from build123d import *

# Parameters (mm, degrees)
BOSS_EXTRUDE1_DEPTH                 = 31.75
F_3_32_0_09375_DIAMETER_HOLE1_D     = 2.38125
F_3_32_0_09375_DIAMETER_HOLE1_DEPTH = 25.4
F_3_32_0_09375_DIAMETER_HOLE1_TIP   = 0.715399675
F_10_CLEARANCE_HOLE1_D              = 5.6134
F_10_CLEARANCE_HOLE1_DEPTH          = 25.4
F_10_CLEARANCE_HOLE1_TIP            = 1.686435499
FILLET1_R                           = 2.54


with BuildPart() as part:
    # Sketch1 → Boss-Extrude1 (new body)
    with BuildSketch(Plane.XY):
        Polygon((0, 0), (0, 19.05), (-3.175, 19.05), (-3.175, 3.175), (-19.05, 3.175), (-19.05, 0), align=None)
    extrude(amount=BOSS_EXTRUDE1_DEPTH)

    # 3/32 (0.09375) Diameter Hole1
    with Locations(Plane(origin=(0, 0, 0), x_dir=(0, 0, -1), z_dir=(1, 0, 0))):
        with Locations((-3.175, 0.0889)):
            Hole(F_3_32_0_09375_DIAMETER_HOLE1_D / 2, depth=F_3_32_0_09375_DIAMETER_HOLE1_DEPTH)
            with Locations((0, 0, -(F_3_32_0_09375_DIAMETER_HOLE1_DEPTH + F_3_32_0_09375_DIAMETER_HOLE1_TIP / 2))):  # 118° drill point
                Cone(0, F_3_32_0_09375_DIAMETER_HOLE1_D / 2, F_3_32_0_09375_DIAMETER_HOLE1_TIP, mode=Mode.SUBTRACT)

    # #10 Clearance Hole1
    with Locations(Plane(origin=(0, 3.175, 0), x_dir=(1, 0, 0), z_dir=(0, 1, 0))):
        with Locations((-11.1125, -26.9875), (-11.1125, -4.7625)):
            Hole(F_10_CLEARANCE_HOLE1_D / 2, depth=F_10_CLEARANCE_HOLE1_DEPTH)
            with Locations((0, 0, -(F_10_CLEARANCE_HOLE1_DEPTH + F_10_CLEARANCE_HOLE1_TIP / 2))):  # 118° drill point
                Cone(0, F_10_CLEARANCE_HOLE1_D / 2, F_10_CLEARANCE_HOLE1_TIP, mode=Mode.SUBTRACT)

    # Fillet1
    fillet1_edges = [part.edges().sort_by_distance(p)[0] for p in [
        (-1.5875, 19.05, 31.75),
        (-19.05, 1.5875, 31.75),
        (-19.05, 1.5875, 0),
        (-1.5875, 19.05, 0),
    ]]
    fillet(fillet1_edges, radius=FILLET1_R)


solid = part.part
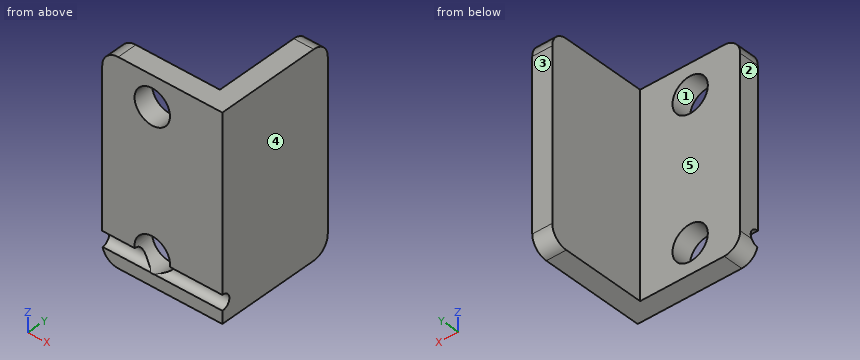
Source: CAD feature listing. Evaluate the final solid. Frame: model axes, mm. Face numbers are marked on the shaded views. A direction names the side the tool comes from. Give positions to 0.01 mm unless a question says otherwise; leave off trailing zeros. Write each loop counter-clockwise with the first axis right and the second up, starting at its lowest first coordinate (ties: lowest second). Pieces come first, ordered by that corner, then holes. Notation, with made-up numbers: (-12, -33.5) -> (-7, -33.5) arc R32 cw to (-7, -3.5) -> close; hole circle Ø2 at (26, 88). An arc over 180 degrees is marked (long way). Write item = value, one per line.
Q1. Cut plane B-B on z = 4. Return loops of the section in (x, y) (3 decimals), then the cut area to 3 significant figures.
Here are the results:
outline = (-19.05, 0.947) -> (-13.814, 0.947) -> (-13.814, 3.175) -> (-19.05, 3.175) -> close; (-8.411, 0.947) -> (0, 0.947) -> (0, 19.05) -> (-3.175, 19.05) -> (-3.175, 3.175) -> (-8.411, 3.175) -> close
area = 80.8 mm²
Q2. Reachability of the marked faces 4 and 5 from +Z, -Z, +X, -X, +Y, -Y: full face, straight path, thin tool, end or side. Return the list, or none.
Here are the results:
face_4 = +Z, -Z, +X, +Y, -Y
face_5 = +Z, -Z, -X, +Y
Q3. Cut plane A-A on x = -12.75. Return loops of the section in (y, z) (3 decimals), then the cut area to 3 significant figures.
Here are the results:
outline = (0, 0) -> (3.175, 0) -> (3.175, 2.483) -> (1.058, 2.483) arc R1.191 cw to (0, 1.988) -> close; (0, 7.042) -> (3.175, 7.042) -> (3.175, 24.708) -> (0, 24.708) -> close; (0, 29.267) -> (3.175, 29.267) -> (3.175, 31.75) -> (0, 31.75) -> close
area = 71.5 mm²
Q4. First-contact query: pin 1 (1 mm diameter, centred on y = 6, z = 16, fed in from -X) (3 decimals); pin 2 (8 mm diameter, centred on y = 5, z = 19.5, fed in from +X); pin 3 (8 mm diameter, centred on x = -13, z = 21, fed in from +Y) (3 decimals). Flat tips, straight axial feed; report the tip coordinate or a pass-through.
Here are the results:
pin_1 = -3.175
pin_2 = 0
pin_3 = 3.175
Q5. Line query: line 1 (X direction, y = 13.5, z = 5) (3 decimals); line 2 (Y direction, x = -5.5, z = 7.5) (3 decimals); line 3 (X direction, y = 2.5, z = 30). Output: solid intervals per line, ascending. Write a range as from..to.
Here are the results:
line_1 = -3.175..0
line_2 = 0..3.175
line_3 = -18.92..0
Q6. Mould query, pull axis X, two halves, no side actions, for the marked faces 1, 2 and 3. Classes: +X half, -X half, draft (parallel to the pull), parting line (faces both ways), or undercut.
Here are the results:
face_1 = undercut
face_2 = -X half
face_3 = draft
Q7. Cut plane C-C on x = -14.75. Return loops of the section in (y, z) (3 decimals).
Here are the results:
outline = (0, 0) -> (3.175, 0) -> (3.175, 31.75) -> (0, 31.75) -> (0, 4.362) arc R1.191 cw (long way) to (0, 1.988) -> close
Q8. Cut plane D-D on y = 2.25. Return loops of the section in (x, z).
Here are the results:
outline = (-19.05, 2.54) arc R2.54 ccw to (-16.51, 0) -> (0, 0) -> (0, 31.75) -> (-16.51, 31.75) arc R2.54 ccw to (-19.05, 29.21) -> close; hole circle Ø5.61 at (-11.11, 4.76); hole circle Ø5.61 at (-11.11, 26.99)
